The listing builds one solid part. Answer for the finished solid, in the listing's coordinates (mm). Face numbers are marked on the shaded views. Round coordinates to 2 decimals unless told otherwise and drop trailing zeros. Write each loop counter-clockwise with the first axis right and the second up, starting at its lowest first coordinate (ties: lowest second). Pieces come first, ordered by that corner, then holes.
Item 1: Each of these flat-tipped pins is pushed along its axis until it touches: pin 1 (10 mm diameter, centred on x = 14, y = 13, fed in from -Z); pin 2 (2 mm diameter, centred on y = -8.5, z = 7, fed in from +X); pin 3 (1.5 mm diameter, centred on x = -3, z = 8.5, fed in from -Y); pin 4 (1 mm diameter, centred on y = -7, z = 2, fed in from -X). Where does it stop, or does it pass through?
Item 2: Find section B-B on y = 7. Give the vertices of the cut face in (x, z).
Item 3: Find section C-C on z = 7.75. Give the vertices of the cut face in (x, y) (3 decimals), then the cut area to 3 significant figures.
Item 4: For a pull along X with two mould halves and no side action, classify the marked faces 1, 2 and 3 as +X half, -X half, draft (parallel to the pull), parting line (faces both ways), or undercut.
Item 5: Find the intervals of material crossed by probe 1 along Y at (x, z) = (0, 6.25); probe 2 along Y at (x, z) = (-1, 7.75); probe 3 along X at (y, z) = (20, 0.75), in increasing order.
Item 6: Find section A-A on x = 0. Give the vertices of the cut face in (y, z).
Item 7: Find section D-D on y = -9. Give the vertices of the cut face in (x, z), then the cut area to 3 significant figures.
```python
from build123d import *
from build123d.topology import SkipClean

# Parameters (mm, degrees)
ESQUISSE1_R                                = 19.45
ESQUISSE1_R_2                              = 17.55
BOSS_EXTRU_1_DEPTH                         = 15
ESQUISSE1_5_R                              = 1.5
ENL_V_MAT_EXTRU_1_DEPTH                    = 15
BOSS_EXTRU_2_DEPTH                         = 15
R_P_TITION_CIRCULAIRE1_COUNT               = 2
R_P_TITION_CIRCULAIRE1_ANGLE               = 120
R_P_TITION_CIRCULAIRE1_THE_OTHER_WAY_COUNT = 2
R_P_TITION_CIRCULAIRE1_THE_OTHER_WAY_ANGLE = 120


with BuildPart() as part:
    # Esquisse1 → Boss.-Extru.1 (new body)
    with BuildSketch(Plane.XY):
        Circle(ESQUISSE1_R)
        Circle(ESQUISSE1_R_2, mode=Mode.SUBTRACT)
    extrude(amount=BOSS_EXTRU_1_DEPTH)

    # Esquisse1<5> → Enlèv. mat.-Extru.1 (cut)
    with BuildSketch(Plane.XY):
        with Locations((0, 19.45)):
            Circle(ESQUISSE1_5_R)
    enl_v_mat_extru_1 = extrude(amount=ENL_V_MAT_EXTRU_1_DEPTH, mode=Mode.SUBTRACT)

    # Esquisse1<6> → Boss.-Extru.2 (add)
    with SkipClean():  # the faces are left unmerged after this step: merging them gives an invalid solid
        with BuildSketch(Plane.XY):
            with BuildLine():
                ThreePointArc((-1.498884406, 19.392159383), (-0.028925687, 20.949721076), (1.5, 19.45))
                ThreePointArc((1.5, 19.45), (1.499721076, 19.421074313), (1.498884406, 19.392159383))
                ThreePointArc((1.498884406, 19.392159383), (2.744536924, 19.255389299), (3.978796705, 19.038688946))
                ThreePointArc((3.978796705, 19.038688946), (3.994695659, 19.244071394), (4, 19.45))
                ThreePointArc((4, 19.45), (-0.205928606, 23.444695659), (-3.978796705, 19.038688946))
                ThreePointArc((-3.978796705, 19.038688946), (-2.744536924, 19.255389299), (-1.498884406, 19.392159383))
            make_face()
        boss_extru_2 = extrude(amount=BOSS_EXTRU_2_DEPTH)

    # Répétition circulaire1: Enlèv. mat.-Extru.1, Boss.-Extru.2 ×2 about axis
    with SkipClean():  # the faces are left unmerged after this step: merging them gives an invalid solid
        r_p_tition_circulaire1_axis = Axis((0, 0, 15), (0, 0, -1))
        add([enl_v_mat_extru_1.rotate(r_p_tition_circulaire1_axis, i * R_P_TITION_CIRCULAIRE1_ANGLE / (R_P_TITION_CIRCULAIRE1_COUNT - 1)) for i in range(1, R_P_TITION_CIRCULAIRE1_COUNT)], mode=Mode.SUBTRACT)
        add([boss_extru_2.rotate(r_p_tition_circulaire1_axis, i * R_P_TITION_CIRCULAIRE1_ANGLE / (R_P_TITION_CIRCULAIRE1_COUNT - 1)) for i in range(1, R_P_TITION_CIRCULAIRE1_COUNT)])

    # Répétition circulaire1 the other way: Enlèv. mat.-Extru.1, Boss.-Extru.2 ×2 about axis
    with SkipClean():  # the faces are left unmerged after this step: merging them gives an invalid solid
        r_p_tition_circulaire1_the_other_way_axis = Axis((0, 0, 15), (0, 0, 1))
        add([enl_v_mat_extru_1.rotate(r_p_tition_circulaire1_the_other_way_axis, i * R_P_TITION_CIRCULAIRE1_THE_OTHER_WAY_ANGLE / (R_P_TITION_CIRCULAIRE1_THE_OTHER_WAY_COUNT - 1)) for i in range(1, R_P_TITION_CIRCULAIRE1_THE_OTHER_WAY_COUNT)], mode=Mode.SUBTRACT)
        add([boss_extru_2.rotate(r_p_tition_circulaire1_the_other_way_axis, i * R_P_TITION_CIRCULAIRE1_THE_OTHER_WAY_ANGLE / (R_P_TITION_CIRCULAIRE1_THE_OTHER_WAY_COUNT - 1)) for i in range(1, R_P_TITION_CIRCULAIRE1_THE_OTHER_WAY_COUNT)])


solid = part.part
```
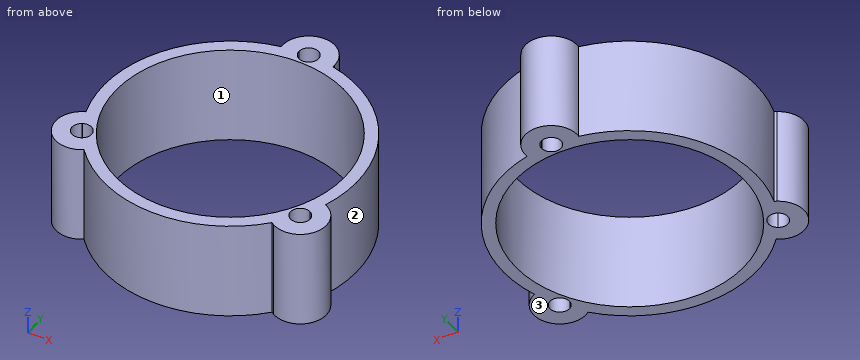
Check values:
1. pin 1: stops at z = 0
1. pin 2: stops at x = 20.84
1. pin 3: stops at y = -19.32
1. pin 4: stops at x = -20.17
2. outline: (-18.15, 0) - (-16.09, 0) - (-16.09, 15) - (-18.15, 15) - close; (16.09, 0) - (18.15, 0) - (18.15, 15) - (16.09, 15) - close
3. outline: (-18.477, -6.074) arc R4 ccw (long way) to (-14.499, -12.965) arc R19.45 ccw to (14.499, -12.965) arc R4 ccw (long way) to (18.477, -6.074) arc R19.45 ccw to (3.979, 19.039) arc R4 ccw (long way) to (-3.979, 19.039) arc R19.45 ccw to start; hole (-17.594, -8.426) arc R1.5 ccw (long way) to (-17.544, -8.398) arc R1.5 ccw to start; hole circle Ø35.1 at (0, 0); hole (1.499, 19.392) arc R1.5 ccw to (1.5, 19.45) arc R1.5 ccw (long way) to start; hole (16.045, -10.994) arc R1.5 ccw to (16.094, -11.024) arc R1.5 ccw (long way) to start
3. area: 278 mm2
4. face 1: undercut
4. face 2: +X half
4. face 3: draft
5. probe 1: y = -19.45 to -17.55, 17.55 to 17.95, 20.95 to 23.45
5. probe 2: y = -19.42 to -17.52, 17.52 to 18.33, 20.57 to 23.32
5. probe 3: x = -3.96 to -1.4, 1.4 to 3.96
6. outline: (-19.45, 0) - (-17.55, 0) - (-17.55, 15) - (-19.45, 15) - close; (17.55, 0) - (17.95, 0) - (17.95, 15) - (17.55, 15) - close; (20.95, 0) - (23.45, 0) - (23.45, 15) - (20.95, 15) - close
7. outline: (-20.78, 0) - (-18.16, 0) - (-18.16, 15) - (-20.78, 15) - close; (-15.53, 0) - (-15.07, 0) - (-15.07, 15) - (-15.53, 15) - close; (15.07, 0) - (15.53, 0) - (15.53, 15) - (15.07, 15) - close; (18.16, 0) - (20.78, 0) - (20.78, 15) - (18.16, 15) - close
7. area: 92.6 mm2
